Read the model definition and answer for the solid it produces. Units are mm, in the model's axes. Face numbers are marked on the shaded views. A direction names the side the tool comes from. Give positions to 0.01 mm unless a question says otherwise; leave off trailing zeros. Order: outer loops, then holes, each group sorted by start corner. A loop starts at its lowest first (then second) coordinate and runs counter-clockwise, first axis right, second up.
```python
from build123d import *

# Parameters (mm, degrees)
BOSS_EXTRUDE1_DEPTH = 16
SKETCH3_R           = 2.25
CUT_EXTRUDE1_DEPTH  = 46.343136195
SKETCH2_R           = 2.5
CUT_EXTRUDE2_DEPTH  = 46.343136195
SKETCH4_R           = 5
CUT_EXTRUDE3_DEPTH  = 40.446165923
SKETCH5_R           = 4
CUT_EXTRUDE4_DEPTH  = 40.446165847
CHAMFER1_SIZE       = 3
FILLET2_R           = 4


with BuildPart() as part:
    # Sketch1 → Boss-Extrude1 (new body)
    with BuildSketch(Plane.XY):
        Polygon((0, 0), (10, 0), (30, 20), (30, 30), (0, 30), align=None)
    extrude(amount=BOSS_EXTRUDE1_DEPTH)

    # Sketch3 → Cut-Extrude1 (cut, through all)
    with BuildSketch(Plane(origin=(0, 30, 0), x_dir=(1, 0, 0), z_dir=(0, 1, 0))):
        with Locations(Location((20, -8, 0), (0, 0, 180))):
            Circle(SKETCH3_R)
    extrude(amount=-CUT_EXTRUDE1_DEPTH, mode=Mode.SUBTRACT)

    # Sketch2 → Cut-Extrude2 (cut, through all)
    with BuildSketch(Plane.ZY):
        with Locations(Location((8, 10, 0), (0, 0, 270))):
            Circle(SKETCH2_R)
    extrude(amount=-CUT_EXTRUDE2_DEPTH, mode=Mode.SUBTRACT)

    # Sketch4 → Cut-Extrude3 (cut, through all)
    with BuildSketch(Plane.ZY.offset(-10)):
        with Locations(Location((8, 10, 0), (0, 0, 270))):
            Circle(SKETCH4_R)
    extrude(amount=-CUT_EXTRUDE3_DEPTH, mode=Mode.SUBTRACT)

    # Sketch5 → Cut-Extrude4 (cut, through all)
    with BuildSketch(Plane(origin=(0, 20, 0), x_dir=(1, 0, 0), z_dir=(0, 1, 0))):
        with Locations(Location((20, -8, 0), (0, 0, 180))):
            Circle(SKETCH5_R)
    extrude(amount=-CUT_EXTRUDE4_DEPTH, mode=Mode.SUBTRACT)

    # Chamfer1
    # the kernel refuses this chamfer: 3 mm, written as the material it adds along each edge
    with BuildSketch(Plane(origin=(10, 10, 8), x_dir=(0, -1, 0), z_dir=(0, 0, -1))) as chamfer1_piece_1_section:
        Polygon((5, -CHAMFER1_SIZE), (5 - CHAMFER1_SIZE, 0), (5, 0), align=None)
    chamfer1_piece_1 = revolve(axis=Axis((10, 10, 8), (-1, 0, 0)), mode=Mode.PRIVATE)
    chamfer1_piece_1 = chamfer1_piece_1 - Plane(origin=(11.757355127, 10, 8), x_dir=(0, -1, 0), z_dir=(-1, 0, 0)) * Cylinder(2.5, 21, mode=Mode.PRIVATE)
    add(chamfer1_piece_1)

    # Fillet2
    fillet2_edges = [part.edges().sort_by_distance(p)[0] for p in [
        (30, 20, 8),
        (10, 0, 8),
    ]]
    fillet(fillet2_edges, radius=FILLET2_R)


solid = part.part
```
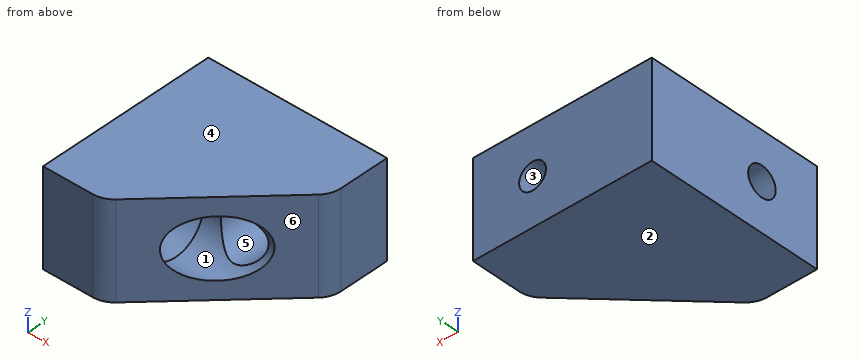
1) Consider L1, parallel to Z at x = 20, y = 15; L2, parallel to Z at x = 20, y = 24; L3, parallel to Y at x = 17, z = 8. Determine where each line is inside the solid, lowest interval first.
Final values:
L1: z = 0 to 4, 12 to 16
L2: z = 0 to 5.75, 10.25 to 16
L3: y = 20 to 30
2) A tool of negligible diameter and unlimited length cuts with its end or side. For the marked faces 1 and 2, from which of +Z, -Z, +X, -X, +Y, -Y can it reach the whole face along a straight path? Write none if from no direction.
Final values:
face 1: +X
face 2: -Z, +X, -X, +Y, -Y
3) Given pin 1 (6 mm diameter, centred on x = 23.5, y = 7, fed in from -Z); pin 2 (1.5 mm diameter, centred on y = 12, z = 8, fed in from +X); pin 3 (3 mm diameter, centred on x = 16, z = 5, fed in from -Y); pin 4 (6.5 mm diameter, centred on x = 20, z = 7, fed in from -Y), each flat-ended and moving along its own axis, determine where each tip first touches the part or whether it passes through.
Final values:
pin 1: passes through
pin 2: stops at x = 10.75
pin 3: stops at y = 4.5
pin 4: stops at y = 12.63
4) The part is cut by section B-B on x = 20. Determine the outline of the cut face in (y, z).
Final values:
outline: (10, 0) - (30, 0) - (30, 5.75) - (20, 5.75) - (20, 4) - (13, 4) arc R5 cw to (10, 3) - close; (10, 13) arc R5 cw to (13, 12) - (20, 12) - (20, 10.25) - (30, 10.25) - (30, 16) - (10, 16) - close
5) The part is cut by section C-C on z = 8. Determine the outline of the cut face in (x, y).
Final values:
outline: (0, 0) - (8.34, 0) arc R4 ccw to (11.17, 1.17) - (15, 5) - (13, 5) - (10.5, 7.5) - (0, 7.5) - close; (0, 12.5) - (10.5, 12.5) - (13, 15) - (16, 15) - (16, 20) - (17.75, 20) - (17.75, 30) - (0, 30) - close; (22.25, 20) - (24, 20) - (24, 15) - (25, 15) - (28.83, 18.83) arc R4 ccw to (30, 21.66) - (30, 30) - (22.25, 30) - close
6) For a pull along X with two mould halves and no side action, classify the marked faces 3, 4, 5 and 6 as released by +X, released by -X, zero draft, split by the parting line, or undercut.
Final values:
face 3: undercut
face 4: zero draft
face 5: undercut
face 6: released by +X
7) The part is cut by section A-A on y = 10. Determine the outline of the cut face in (x, z), and give its area (3 significant figures).
Final values:
outline: (0, 0) - (20, 0) - (20, 3) - (13, 3) - (10.5, 5.5) - (0, 5.5) - close; (0, 10.5) - (10.5, 10.5) - (13, 13) - (20, 13) - (20, 16) - (0, 16) - close
area: 179 mm2
8) The part is cut by section D-D on x = 7. Determine the outline of the cut face in (y, z), and give its area (3 significant figures).
Final values:
outline: (0, 0) - (30, 0) - (30, 16) - (0, 16) - close; hole circle Ø5 at (10, 8)
area: 460 mm2
